For this review, take the finished solid that the model builds, in its own axes (mm). A direction names the side the tool comes from. Coordinates: 2 decimals unless noted, no trailing zeros. Order: outer loops, then holes, each group sorted by start corner. A loop starts at its lowest first (then second) coordinate and runs counter-clockwise, first axis right, second up.
Autodesk Inventor part; units mm, degrees
ref_plane "YZ Plane" through (0, 0, 0) normal (1, 0, 0) x (0, 1, 0)
ref_plane "XZ Plane" through (0, 0, 0) normal (0, 1, 0) x (-1, 0, 0)
ref_plane "XY Plane" through (0, 0, 0) normal (0, 0, 1) x (1, 0, 0)
sketch "スケッチ1" plane through (0, 0, 0) normal (0, 0, 1) x (1, 0, 0)
  line L0 (1.2, -2.75) -> (1.2, 2.75)
  line L1 (1.2, 2.75) -> (2.7, 2.75)
  line L2 (2.7, 2.75) -> (3, 2.45)
  line L3 (3, 2.45) -> (3, -2.45)
  line L4 (0, 6.6667) -> (0, -6.6667) construction
  line L5 (3, -2.45) -> (2.7, -2.75)
  line L6 (2.7, -2.75) -> (1.2, -2.75)
  point P0 (0, 0)
  point P1 (0, 0)
  point P2 (1.2, 0)
  point P3 (3, 0)
  dimension "d0" = 6
  dimension "d1" = 2.4
  dimension "d3" = 5.5
  dimension "d4" = 0.3
  dimension "d5" = 0.3
revolve "回転1" add sketch "スケッチ1" angle 360 about axis through (0, 6.6667, 0) along (0, -1, 0)
sketch "スケッチ2" plane through (0, -2.75, 0) normal (0, -1, 0) x (1, 0, 0)
  line L0 (-0.5, 3) -> (0.5, 3)
  line L1 (0.5, 3) -> (0.5, -3)
  line L2 (0.5, -3) -> (-0.5, -3)
  line L3 (-0.5, -3) -> (-0.5, 3)
  line L4 (-0.5, 3) -> (0.5, -3) construction
  line L5 (0.5, 3) -> (-0.5, -3) construction
  point P0 (0, 0)
  dimension "d7" = 1
  dimension "d8" = 6
extrude "押し出し1" cut sketch "スケッチ2" against normal blind 1
equation "\"d5\" = d4"
properties part number "ARU-304S" material "ステンレス鋼 440C"
1. Take a section at B-B, the plane z = 0. Give the boundary of the cut face in (x, y).
Answer below:
outline: (-3, -2.45) - (-2.7, -2.75) - (-1.2, -2.75) - (-1.2, 2.75) - (-2.7, 2.75) - (-3, 2.45) - close; (1.2, -2.75) - (2.7, -2.75) - (3, -2.45) - (3, 2.45) - (2.7, 2.75) - (1.2, 2.75) - close
2. Clearance check with flat-ended pins moving along their axes: pin 1 Ø0.8 at (x, z) = (0, -2) entering from -Y; pin 2 Ø0.8 at (y, z) = (-2.5, 1.5) entering from +X; pin 3 Ø0.8 at (y, z) = (-2.5, 2) entering from -X. State where each tip first meets the part, or that it passes through.
Answer below:
pin 1: stops at y = -1.75
pin 2: stops at x = 2.79
pin 3: stops at x = -2.54
3. The part is to be moulded in two halves that separate along X. For faces 1 (the face through (1, 2.75, -1)), 2 (the face through (0.5, -2, -2)), 3 (the face through (2.82, -2.63, 0.06)), say which applies: +X half, -X half, draft (parallel to the pull), parting line (faces both ways), or undercut.
Answer below:
face 1: draft
face 2: undercut
face 3: +X half
4. To check wall thickness, follow L1, parallel to Z at x = 0, y = 1.6; L2, parallel to X at y = -0.75, z = 0.5. State the ranges of each line that lie inside material, in increasing order.
Answer below:
L1: z = -3 to -1.2, 1.2 to 3
L2: x = -2.96 to -1.09, 1.09 to 2.96
5. Machinability: for faces 4 (the face through (2, -2.75, 0)), 5 (the face through (-0.5, -2, -2)), which of the approach directions +Z, -Z, +X, -X, +Y, -Y give a long, thin tool a straight path to every point of the face, cutting with its end or side? Answer none if there is none.
Answer below:
face 4: +Z, -Z, +X, -X, -Y
face 5: +Z, -Z, -Y
6. Take a section at C-C, the plane y = 0.65. Give the boundary of the cut face in (x, z), plus the area to 3 significant figures.
Answer below:
outline: circle Ø6 at (0, 0); hole circle Ø2.4 at (0, 0)
area: 23.8 mm2
7. Take a section at A-A, the plane x = 0. Give the boundary of the cut face in (y, z), plus the area to 3 significant figures.
Answer below:
outline: (-1.75, -3) - (2.45, -3) - (2.75, -2.7) - (2.75, -1.2) - (-1.75, -1.2) - close; (-1.75, 1.2) - (2.75, 1.2) - (2.75, 2.7) - (2.45, 3) - (-1.75, 3) - close
area: 16.1 mm2
